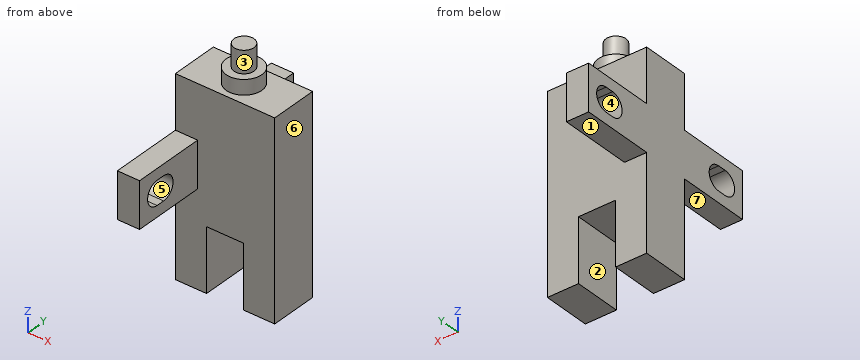
from build123d import *

# Parameters (mm, degrees)
SKETCH1_W           = 13.4
SKETCH1_H           = 26.2
BOSS_EXTRUDE1_DEPTH = 6.4
SKETCH2_W           = 5
SKETCH2_H           = 8.5
CUT_EXTRUDE1_DEPTH  = 6.4
SKETCH3_W           = 6.2
SKETCH3_H           = 26
BOSS_EXTRUDE2_DEPTH = 3
CUT_EXTRUDE2_DEPTH  = 4


with BuildPart() as part:
    # Sketch1 → Boss-Extrude1 (new body)
    with BuildSketch(Plane(origin=(0, 0, 0), x_dir=(1, 0, 0), z_dir=(0, 1, 0))):
        with Locations((0, 13.1)):
            Rectangle(SKETCH1_W, SKETCH1_H)
    extrude(amount=BOSS_EXTRUDE1_DEPTH)

    # Sketch2 → Cut-Extrude1 (cut)
    with BuildSketch(Plane(origin=(0, 6.4, 0), x_dir=(1, 0, 0), z_dir=(0, 1, 0))):
        with Locations((0, 21.95)):
            Rectangle(SKETCH2_W, SKETCH2_H)
    extrude(amount=-CUT_EXTRUDE1_DEPTH, mode=Mode.SUBTRACT)

    # Sketch3 → Boss-Extrude2 (add)
    with BuildSketch(Plane.ZY.offset(6.7)):
        with Locations((-10.3, 3.2)):
            Rectangle(SKETCH3_W, SKETCH3_H)
    extrude(amount=-BOSS_EXTRUDE2_DEPTH)

    # Sketch4 → Cut-Extrude2 (cut, through all)
    with BuildSketch(Plane(origin=(-3.7, 0, 0), x_dir=(0, 0, -1), z_dir=(1, 0, 0))):
        with BuildLine():
            Line((11.9, 13.25), (11.9, 12.15))
            ThreePointArc((11.9, 12.15), (10.3, 10.55), (8.7, 12.15))
            Line((8.7, 12.15), (8.7, 13.25))
            ThreePointArc((8.7, 13.25), (10.3, 14.85), (11.9, 13.25))
        make_face()
        with BuildLine():
            Line((11.9, -6.85), (11.9, -5.75))
            ThreePointArc((11.9, -5.75), (10.3, -4.15), (8.7, -5.75))
            Line((8.7, -5.75), (8.7, -6.85))
            ThreePointArc((8.7, -6.85), (10.3, -8.45), (11.9, -6.85))
        make_face()
    extrude(amount=-CUT_EXTRUDE2_DEPTH, mode=Mode.SUBTRACT)

    # Sketch5 → Revolve1 (revolve)
    with BuildSketch(Plane(origin=(0, 0, 0), x_dir=(0, 0, -1), z_dir=(1, 0, 0))):
        Polygon((0, 3.2), (0, 5.6), (-2, 5.6), (-2, 4.55), (-5, 4.55), (-5, 3.2), align=None)
    revolve(axis=Axis((0, 3.2, -27.354495769), (0, 0, 1)))


solid = part.part
Model file for the job. Use its own axes, mm. Face numbers are marked on the shaded views. A direction names the side the tool comes from. Round coordinates to 2 decimals unless told otherwise and drop trailing zeros. Order: outer loops, then holes, each group sorted by start corner. A loop starts at its lowest first (then second) coordinate and runs counter-clockwise, first axis right, second up. Notation, with made-up numbers: M 0.25,23.5 L 10.25,23.5 A15 cw 10.25,48.5 Z; hole C -35,65 d9. An arc over 180 degrees is marked long. Write each question's results on one line, items separated by ' | '. Start each with the question number.
(1) Saw through at C-C, the plane y = -5.25. Give the cut face in (x, z).
(2) Probe probe 1 along X at (y, z) = (1, -22); probe 2 along Y at (x, z) = (-3, -21.5); probe 3 along Z at (x, y) = (-5.5, 3). List the from-to ranges inside material, lowest first. Write a range as from..to.
(3) Saw through at A-A, the plane x = -5.5. Give the cut face in (y, z).
(4) Drop flat-ended pins along their axis: pin 1 (0.9 mm diameter, centred on x = -6, y = -6.5, fed in from +Z); pin 2 (1.2 mm diameter, centred on x = -5.5, y = 12.5, fed in from -Z); pin 3 (5 mm diameter, centred on x = 4.5, y = 3, fed in from +Z); pin 4 (10 mm diameter, centred on y = 11.5, z = -20, fed in from -X). Give the stop position or say it passes through.
(5) Two-plate mould, pull along Z, no slides. Class the marked faces 5, 6 and 7: pulls with the +Z half, pulls with the -Z half, needs draft (parallel to the pull), parting line crosses it, or undercut.
(6) Saw through at D-D, the plane x = 0. Give the cut face in (y, z).
(7) Which spindle directions (+Z, -Z, +X, -X, +Y, -Y) get a long thin tool onto all of the face, cutting with end or side? Do the marked faces 1, 2, 3 and 4. Say none if no direction does.
(8) Saw through at B-B, the plane z = -10.3. Give the cut face in (x, y).
Established:
1) outline: M -6.7,-13.4 L -3.7,-13.4 L -3.7,-11.82 L -6.7,-11.82 Z; M -6.7,-8.78 L -3.7,-8.78 L -3.7,-7.2 L -6.7,-7.2 Z
2) probe 1: x = -6.7..-2.5, 2.5..6.7 | probe 2: y = 0..6.4 | probe 3: z = -26.2..0
3) outline: M -9.8,-13.4 L 0,-13.4 L 0,-26.2 L 6.4,-26.2 L 6.4,-13.4 L 16.2,-13.4 L 16.2,-7.2 L 6.4,-7.2 L 6.4,0 L 0,0 L 0,-7.2 L -9.8,-7.2 Z; hole M -6.85,-11.9 L -5.75,-11.9 A1.6 ccw -5.75,-8.7 L -6.85,-8.7 A1.6 ccw Z; hole M 12.15,-11.9 L 13.25,-11.9 A1.6 ccw 13.25,-8.7 L 12.15,-8.7 A1.6 ccw Z
4) pin 1: stops at z = -7.2 | pin 2: stops at z = -13.4 | pin 3: stops at z = 2 | pin 4: passes through
5) face 5: undercut | face 6: needs draft | face 7: pulls with the -Z half
6) outline: M 0,-17.7 L 6.4,-17.7 L 6.4,0 L 5.6,0 L 5.6,2 L 4.55,2 L 4.55,5 L 1.85,5 L 1.85,2 L 0.8,2 L 0.8,0 L 0,0 Z
7) face 1: -Z, +X, -X, +Y | face 2: -Z, +Y, -Y | face 3: +Z | face 4: +X, -X
8) outline: M -6.7,-9.8 L -3.7,-9.8 L -3.7,-8.45 L -6.7,-8.45 Z; M -6.7,-4.15 L -3.7,-4.15 L -3.7,0 L 6.7,0 L 6.7,6.4 L -3.7,6.4 L -3.7,10.55 L -6.7,10.55 Z; M -6.7,14.85 L -3.7,14.85 L -3.7,16.2 L -6.7,16.2 Z
